Part model, mm, in its own coordinate system. A direction names the side the tool comes from. Round coordinates to 2 decimals unless told otherwise and drop trailing zeros. Write each loop counter-clockwise with the first axis right and the second up, starting at its lowest first coordinate (ties: lowest second). Pieces come first, ordered by that corner, then holes.
from build123d import *

# Parameters (mm, degrees)
F0_W     = 23.5931184143
F0_H     = 41.4473693818
F1_DEPTH = 25
F2_DEPTH = 25


with BuildPart() as f1:
    # F0 (on Top) → F1 (new body)
    with BuildSketch(Plane.XY):
        Polygon((-2.3911930621, 12.2747989371), (-20.5642711371, 12.2747989371), (-78.9094138891, 12.2747989371), (-78.9094138891, -6.0576931573), (21.2019253522, -6.0576931573), (21.2019253522, 12.2747989371), align=None)
        with Locations((9.4053661451, 32.998483628)):
            Rectangle(F0_W, F0_H)
        Polygon((-78.9094138891, 53.7221683189), (-20.5642711371, 53.7221683189), (-2.3911930621, 53.7221683189), (21.2019253522, 53.7221683189), (21.2019253522, 72.2140744328), (-78.9094138891, 72.2140744328), align=None)
        Polygon((-78.9094138891, 12.2747989371), (-20.5642711371, 12.2747989371), (-49.7368425131, 32.998483628), align=None)
    extrude(amount=F1_DEPTH)

    # F0 (on Top) → F2 (join)
    with BuildSketch(Plane.XY):
        Polygon((-78.9094138891, 53.7221683189), (-49.7368425131, 32.998483628), (-20.5642711371, 53.7221683189), align=None)
        Polygon((-49.7368425131, 32.998483628), (-20.5642711371, 12.2747989371), (-2.3911930621, 12.2747989371), (-2.3911930621, 53.7221683189), (-20.5642711371, 53.7221683189), align=None)
    extrude(amount=F2_DEPTH)


solid = f1.part
Q1. Saw through at C-C, the plane y = 43.5. Write the cut outline in (x, z), and give its area (3 significant figures).
Q2. Tool access for faces 1 (the flat face through (21.202, 33, 12)), 2 (the flat face through (-64.12, 22.78, 12.32)): list every direction of +Z, -Z, +X, -X, +Y, -Y with a clear straight run to the whole face (end or side of a thin tool).
Q3. Saw through at A-A, the plane z = 15. Write the cut outline in (x, y), and give its area (3 significant figures).
Q4. Saw through at B-B, the plane x = -62. Write the cut outline in (y, z).
Q5. Saw through at D-D, the plane y = 24. Write the cut outline in (x, z).
Q6. Wall check: line 1 (Y direction, x = -60.5, z = 21); line 2 (Y direction, x = -64.5, z = 7.75); line 3 (X direction, y = 19, z = 15.25). Give the ranges that are in metal, low to high.
Q7. Drop a flat-ended pin along its axis: P1, Ø8, axis at y = 31, z = 10, coming from the -X side. Give the stop position or say it passes through.
Q8. Two-plate mould, pull along Y, no slides. Class faces 3 (the flat face through (-30, -6.058, 12)), 4 (the flat face through (-64.527, 43.505, 12.325)), 5 (the flat face through (-28, 72.214, 12)), 6 (the flat face through (-30, 34, 25)): released by +Y, released by -Y, zero draft, split by the parting line, or undercut.
Computed:
1. outline: (-64.52, 0) - (21.2, 0) - (21.2, 25) - (-64.52, 25) - close
1. area: 2,140 mm2
2. face 1: +Z, -Z, +X, +Y, -Y
2. face 2: +Z, -Z, -X
3. outline: (-78.91, -6.06) - (21.2, -6.06) - (21.2, 72.21) - (-78.91, 72.21) - (-78.91, 53.72) - (-49.74, 33) - (-78.91, 12.27) - close
3. area: 7,230 mm2
4. outline: (-6.06, 0) - (24.29, 0) - (24.29, 25) - (-6.06, 25) - close; (41.71, 0) - (72.21, 0) - (72.21, 25) - (41.71, 25) - close
5. outline: (-62.4, 0) - (21.2, 0) - (21.2, 25) - (-62.4, 25) - close
6. line 1: y = -6.06 to 25.35, 40.64 to 72.21
6. line 2: y = -6.06 to 22.51, 43.49 to 72.21
6. line 3: x = -69.44 to 21.2
7. P1: stops at x = -58.18
8. face 3: released by -Y
8. face 4: undercut
8. face 5: released by +Y
8. face 6: zero draft
